Input: part model. Units: mm. Frame: model coordinates. Face numbers are marked on the shaded views. Round coordinates to 2 decimals unless told otherwise and drop trailing zeros. Loops run counter-clockwise (first coordinate to the right, second up) from the corner with the lowest first, then second, coordinate; pieces in that order, holes last. Notation, with made-up numbers: M 36,32.25 L 77,32.25 A19 cw 77,59.25 Z; hole C -25,60.5 d5. An arc over 180 degrees is marked long. Use one line per item in the form item = value. Start each with the question number.
Q1. Section query A-A, the plane z = 0. Output: boundary loops of the cut face in (x, y).
Q2. Section query D-D, the plane z = -2.1. Output: boundary loops of the cut face in (x, y), and give its area (3 significant figures).
Q3. Mould query, pull axis X, two halves, no side actions, for the marked faces 1, 2 and 3. Classes: pulls with the +X half, pulls with the -X half, needs draft (parallel to the pull), parting line crosses it, or undercut.
Q4. Ray query, line 1 along X through (y, z) = (0.35, 0); line 2 along Z through (x, y) = (-0.9, -1.4). Return the intervals inside material, ascending.
Q5. Section query B-B, the plane x = 0. Output: boundary loops of the cut face in (y, z).
Q6. Section query C-C, the plane y = 0.55. Output: boundary loops of the cut face in (x, z).
```python
from build123d import *

# Parameters (mm, degrees)
CROQUIS1_W              = 5
CROQUIS1_H              = 5
SALIENTE_EXTRUIR1_DEPTH = 2.5
CROQUIS2_R              = 1
CORTAR_EXTRUIR1_DEPTH   = 6
REDONDEO1_R             = 0.5


with BuildPart() as part:
    # Croquis1 → Saliente-Extruir1 (new body, symmetric)
    with BuildSketch(Plane(origin=(0, 0, 0), x_dir=(1, 0, 0), z_dir=(0, 1, 0))):
        Rectangle(CROQUIS1_W, CROQUIS1_H)
    extrude(amount=SALIENTE_EXTRUIR1_DEPTH, both=True)

    # Croquis2 → Cortar-Extruir1 (cut, through all)
    with BuildSketch(Plane(origin=(0, 2.5, 0), x_dir=(1, 0, 0), z_dir=(0, 1, 0))):
        Circle(CROQUIS2_R)
    extrude(amount=-CORTAR_EXTRUIR1_DEPTH, mode=Mode.SUBTRACT)

    # Redondeo1
    redondeo1_edges = [part.edges().sort_by_distance(p)[0] for p in [
        (-2.5, 2.5, 0),
        (0, 2.5, 2.5),
        (-1, -2.5, 0),
        (-1, 2.5, 0),
        (2.5, 2.5, 0),
        (0, -2.5, 2.5),
        (-2.5, -2.5, 0),
        (0, -2.5, -2.5),
        (2.5, -2.5, 0),
        (0, 2.5, -2.5),
        (2.5, 0, 2.5),
        (-2.5, 0, 2.5),
        (-2.5, 0, -2.5),
        (2.5, 0, -2.5),
    ]]
    fillet(redondeo1_edges, radius=REDONDEO1_R)


solid = part.part
```
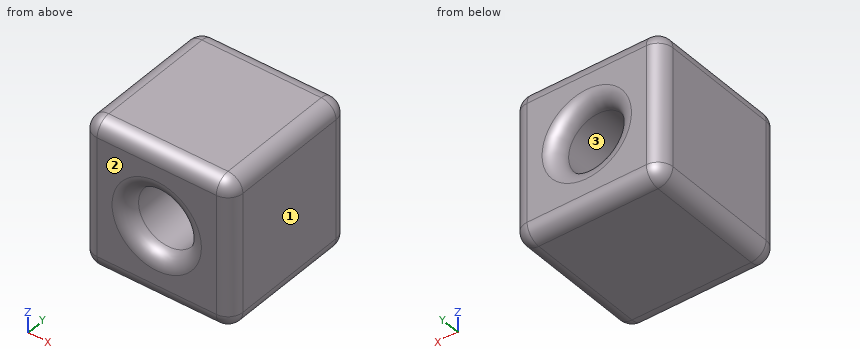
Results found:
q1.outline = M -2.5,-2 A0.5 ccw -2,-2.5 L -1.5,-2.5 A0.5 ccw -1,-2 L -1,2 A0.5 ccw -1.5,2.5 L -2,2.5 A0.5 ccw -2.5,2 Z; M 1,-2 A0.5 ccw 1.5,-2.5 L 2,-2.5 A0.5 ccw 2.5,-2 L 2.5,2 A0.5 ccw 2,2.5 L 1.5,2.5 A0.5 ccw 1,2 Z
q2.outline = M -2.49,-2 A0.49 ccw -2,-2.49 L 2,-2.49 A0.49 ccw 2.49,-2 L 2.49,2 A0.49 ccw 2,2.49 L -2,2.49 A0.49 ccw -2.49,2 Z
q2.area = 24.6 mm²
q3.face_1 = pulls with the +X half
q3.face_2 = needs draft
q3.face_3 = undercut
q4.line_1 = -2.5 to -1, 1 to 2.5
q4.line_2 = -2.5 to -0.44, 0.44 to 2.5
q5.outline = M -2.5,-2 A0.5 ccw -2,-2.5 L 2,-2.5 A0.5 ccw 2.5,-2 L 2.5,-1.5 A0.5 ccw 2,-1 L -2,-1 A0.5 ccw -2.5,-1.5 Z; M -2.5,1.5 A0.5 ccw -2,1 L 2,1 A0.5 ccw 2.5,1.5 L 2.5,2 A0.5 ccw 2,2.5 L -2,2.5 A0.5 ccw -2.5,2 Z
q6.outline = M -2.5,-2 A0.5 ccw -2,-2.5 L 2,-2.5 A0.5 ccw 2.5,-2 L 2.5,2 A0.5 ccw 2,2.5 L -2,2.5 A0.5 ccw -2.5,2 Z; hole C 0,0 d2
